Could you check a few things on this model? Use its own coordinates, in mm. Give positions to 0.01 mm unless a question says otherwise; leave off trailing zeros. Loops run counter-clockwise (first coordinate to the right, second up) from the corner with the lowest first, then second, coordinate; pieces in that order, holes last. Notation, with made-up numbers: M 76.25,84.5 L 130.25,84.5 A17 ccw 130.25,108.5 Z; hole C -39.5,-14 d1. An arc over 180 degrees is marked long. Return JSON: item names as keys, results as strings. Group by question number.
1. If we section it at C-C (z = 4.5): Write out the boundary of the cut face in (x, y) (3 decimals), plus the area to 3 significant figures.
2. If we section it at A-A (x = 85): Write out the boundary of the cut face in (y, z), plus the area to 3 significant figures.
3. For pin 1 (2 mm diameter, centred on x = 35.5, z = 4.5, fed in from -Y); pin 2 (1.5 mm diameter, centred on x = -36, z = 4.5, fed in from +Y), each with a flat end and sliding along its axis, tell me the tip position at first contact or that it passes through.
4. Please list where these lines run through material, in increasing order: line 1 (Y direction, x = 0, z = 4.75); line 2 (Y direction, x = 85, z = 2.75); line 3 (X direction, y = -1.5, z = 0.5).
5. If we section it at D-D (y = 35): Write out the boundary of the cut face in (x, z).
6. If we section it at B-B (x = 0): Write out the boundary of the cut face in (y, z).
```python
from build123d import *

# Parameters (mm, degrees)
SKETCH1_R           = 10.5
SKETCH1_R_2         = 8
BOSS_EXTRUDE2_DEPTH = 7
FILLET4_R           = 6
FILLET5_R           = 6


with BuildPart() as part:
    # Sketch1 → Boss-Extrude2 (new body)
    with BuildSketch(Plane.XY):
        with BuildLine():
            Line((71.771243445, 9), (20.207259422, 9))
            Line((20.207259422, 9), (42.591220317, 47.770157545))
            ThreePointArc((42.591220317, 47.770157545), (-38.960731457, 50.774613779), (-57.165847871, -28.776133117))
            Line((-57.165847871, -28.776133117), (-8.66103197, -15.779306867))
            ThreePointArc((-8.66103197, -15.779306867), (4.846344572, -17.335309178), (15.588457268, -9))
            Line((15.588457268, -9), (71.771243445, -9))
            ThreePointArc((71.771243445, -9), (101, 0), (71.771243445, 9))
        make_face()
        Circle(SKETCH1_R, mode=Mode.SUBTRACT)
        with Locations((85, 0)):
            Circle(SKETCH1_R_2, mode=Mode.SUBTRACT)
        with BuildLine():
            Line((9, 15.588457268), (25.5, 44.167295593))
            ThreePointArc((25.5, 44.167295593), (-31.046832879, 40.461020355), (-49.262217141, -13.1997713))
            Line((-49.262217141, -13.1997713), (-17.386664873, -4.658742812))
            ThreePointArc((-17.386664873, -4.658742812), (-10.957705722, 14.280360125), (9, 15.588457268))
        make_face(mode=Mode.SUBTRACT)
    extrude(amount=BOSS_EXTRUDE2_DEPTH)

    # Fillet4
    fillet4_edges = [part.edges().sort_by_distance(p)[0] for p in [
        (71.771243445, -9, 3.5),
        (15.588457268, -9, 3.5),
        (-8.66103197, -15.779306867, 3.5),
        (-57.165847871, -28.776133117, 3.5),
        (42.591220317, 47.770157545, 3.5),
        (20.207259422, 9, 3.5),
        (71.771243445, 9, 3.5),
    ]]
    fillet(fillet4_edges, radius=FILLET4_R)

    # Fillet5
    fillet5_edges = [part.edges().sort_by_distance(p)[0] for p in [
        (25.5, 44.167295593, 3.5),
        (-49.262217141, -13.1997713, 3.5),
        (-17.386664873, -4.658742812, 3.5),
        (9, 15.588457268, 3.5),
    ]]
    fillet(fillet5_edges, radius=FILLET5_R)


solid = part.part
```
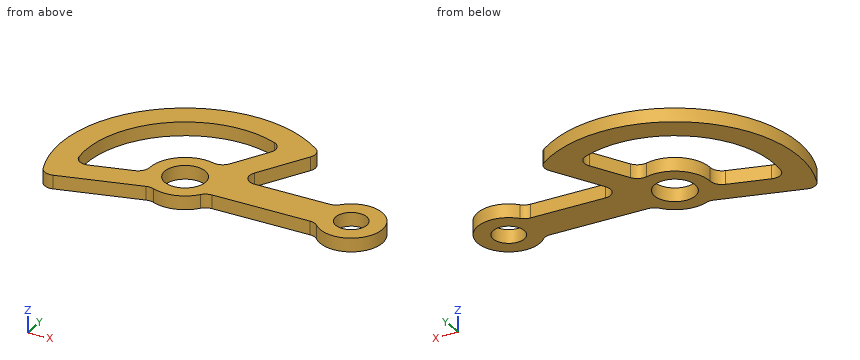
Answer:
{
 "1": {"outline": "M -59.368,-23.904 A6 ccw -52.25,-27.459 L -10.799,-16.352 A6 cw -6.934,-16.611 A18 ccw 14.051,-11.25 A6 cw 18.735,-9 L 68.907,-9 A6 cw 73.296,-10.909 A16 ccw long 73.296,10.909 A6 cw 68.907,9 L 30.6,9 A6 cw 25.403,18 L 40.046,43.362 A6 ccw 38.455,51.158 A64 ccw Z; hole M -50.582,-6.514 A6 ccw -43.079,-11.543 L -22.446,-6.014 A6 ccw -17.999,-0.164 A18 cw 4.817,17.343 A6 ccw 11.619,20.125 L 22.299,38.623 A6 ccw 19.383,47.173 A51 ccw Z; hole C 0,0 d21; hole C 85,0 d16", "area": "5,250 mm²"},
 "2": {"outline": "M -16,0 L -8,0 L -8,7 L -16,7 Z; M 8,0 L 16,0 L 16,7 L 8,7 Z", "area": "112 mm²"},
 "3": {"pin 1": "stops at y = -9", "pin 2": "stops at y = 53.42"},
 "4": {"line 1": "y = -18 to -10.5, 10.5 to 18, 51 to 64", "line 2": "y = -16 to -8, 8 to 16", "line 3": "x = -63.98 to -50.98, -18.14 to -10.39, 10.39 to 77.14, 92.86 to 100.93"},
 "5": {"outline": "M -53.58,0 L -37.09,0 L -37.09,7 L -53.58,7 Z; M 20.21,0 L 35.22,0 L 35.22,7 L 20.21,7 Z"},
 "6": {"outline": "M -18,0 L -10.5,0 L -10.5,7 L -18,7 Z; M 10.5,0 L 18,0 L 18,7 L 10.5,7 Z; M 51,0 L 64,0 L 64,7 L 51,7 Z"}
}
